```python
from build123d import *

# Parameters (mm, degrees)
F1_DEPTH = 7
F2_R     = 1.6
F3_DEPTH = 25
F4_START = -3.9
F2_R_2   = 3.15
F4_DEPTH = 21.1


with BuildPart() as f1:
    # F0 (on Front) → F1 (new body, symmetric)
    with BuildSketch(Plane.XZ):
        Polygon((-75, 0), (0, 0), (0, 6.4), (-2.7, 6.4), (-2.7, 2.5), (-5.7, 2.5), (-5.7, 5.1), (-4.5, 5.1), (-4.5, 6.4), (-4.5, 7.1), (-7.1, 6.4), (-19.2, 6.4), (-19.2, 6.9), (-31.7, 6.9), (-31.2, 6.4), (-28.7, 3.9), (-47.2, 3.9), (-44.7, 6.4), (-44.2, 6.9), (-56.7, 6.9), (-56.7, 6.4), (-68.1, 6.4), (-70.7, 7.1), (-70.7, 6.4), (-70.7, 5.1), (-69.5, 5.1), (-69.5, 2.5), (-72.5, 2.5), (-72.5, 6.4), (-75, 6.4), align=None)
    extrude(amount=F1_DEPTH, both=True)

    # F2 (on face) → F3 (cut)
    with BuildSketch(Plane(origin=(0, 0, 0), x_dir=(1, 0, 0), z_dir=(0, 0, -1))):
        with Locations((-37.5, 0)):
            Circle(F2_R)
        with Locations((-26.5, 0)):
            Circle(F2_R)
    extrude(amount=-F3_DEPTH, mode=Mode.SUBTRACT)

    # F2 (on face) → F4 (cut)
    with BuildSketch(Plane(origin=(0, 0, 0), x_dir=(1, 0, 0), z_dir=(0, 0, -1)).offset(F4_START)):
        with Locations((-26.5, 0)):
            Circle(F2_R_2)
        with Locations((-26.5, 0)):
            Circle(F2_R, mode=Mode.SUBTRACT)
    extrude(amount=-F4_DEPTH, mode=Mode.SUBTRACT)


solid = f1.part
```
Part model, mm, in its own coordinate system. A direction names the side the tool comes from. Round coordinates to 2 decimals unless told otherwise and drop trailing zeros. Loops run counter-clockwise (first coordinate to the right, second up) from the corner with the lowest first, then second, coordinate; pieces in that order, holes last. Notation, with made-up numbers: (9.5, -30.5) -> (22.5, -30.5) arc R29 cw to (22.5, -5.5) -> close; hole circle Ø5 at (37.5, -24). An arc over 180 degrees is marked (long way). Use CSV: the item, a comma, the result in double quotes. Start each with the question number.
1) Pull direction Z, two halves, no side cores. Call faces 1 (the flat face through (-74, 0, 6.4)), 2 (the flat face through (-69.5, 0, 4)), 3 (the cylindrical face through (-27.68, -1.08, 1.92)): +Z half, -Z half, draft (parallel to the pull), parting line (faces both ways), or undercut.
2) Wall check: L1, parallel to X at y = 0, z = 2.2; L2, parallel to Y at x = -37.5, z = 1.4; L3, parallel to X at y = 0.75, z = 4. Give the ranges that are in metal, low to high. Write a range as [from, to].
3) Drop flat-ended pins along their axis: P1, Ø0.8, axis at x = -73.5, y = 1.5, coming from the +Z side; P2, Ø3, axis at x = -27, y = 2.5, coming from the +Z side; P3, Ø5.5, axis at x = -26.5, y = 0, coming from the +Z side. Give the stop position or say it passes through.
4) Which spindle directions (+Z, -Z, +X, -X, +Y, -Y) get a long thin tool onto all of the face, cutting with end or side? Do faces 4 (the flat face through (-38, -2, 0)), 5 (the flat face through (-70, 0, 5.1)), 6 (the flat face through (-62, 0, 6.4)). Say none if no direction does.
5) Cut at C-C, the plane y = -5. Write the cut outline in (x, z), plus the area to 3 significant figures.
6) Cut at B-B, the plane x = -37.5. Write the cut outline in (y, z), plus the area to 3 significant figures.
7) Cut at A-A, the plane z = 5.75. Write the cut outline in (x, y), plus the area to 3 significant figures.
8) Cut at D-D, the plane x = -45. Write the cut outline in (y, z).
Determined:
1,face 1,"+Z half"
1,face 2,"undercut"
1,face 3,"draft"
2,L1,"x = [-75, -39.1], [-35.9, -28.1], [-24.9, 0]"
2,L2,"y = [-7, -1.6], [1.6, 7]"
2,L3,"x = [-75, -72.5], [-69.5, -47.1], [-23.44, -5.7], [-2.7, 0]"
3,P1,"stops at z = 6.4"
3,P2,"stops at z = 6.9"
3,P3,"stops at z = 3.9"
4,face 4,"-Z, +X, -X, +Y, -Y"
4,face 5,"+Y, -Y"
4,face 6,"+Z, +Y, -Y"
5,outline,"(-75, 0) -> (0, 0) -> (0, 6.4) -> (-2.7, 6.4) -> (-2.7, 2.5) -> (-5.7, 2.5) -> (-5.7, 5.1) -> (-4.5, 5.1) -> (-4.5, 7.1) -> (-7.1, 6.4) -> (-19.2, 6.4) -> (-19.2, 6.9) -> (-31.7, 6.9) -> (-28.7, 3.9) -> (-47.2, 3.9) -> (-44.2, 6.9) -> (-56.7, 6.9) -> (-56.7, 6.4) -> (-68.1, 6.4) -> (-70.7, 7.1) -> (-70.7, 5.1) -> (-69.5, 5.1) -> (-69.5, 2.5) -> (-72.5, 2.5) -> (-72.5, 6.4) -> (-75, 6.4) -> close"
5,area,"434 mm2"
6,outline,"(-7, 0) -> (-1.6, 0) -> (-1.6, 3.9) -> (-7, 3.9) -> close; (1.6, 0) -> (7, 0) -> (7, 3.9) -> (1.6, 3.9) -> close"
6,area,"42.1 mm2"
7,outline,"(-75, -7) -> (-72.5, -7) -> (-72.5, 7) -> (-75, 7) -> close; (-70.7, -7) -> (-45.35, -7) -> (-45.35, 7) -> (-70.7, 7) -> close; (-30.55, -7) -> (-4.5, -7) -> (-4.5, 7) -> (-30.55, 7) -> close; (-2.7, -7) -> (0, -7) -> (0, 7) -> (-2.7, 7) -> close; hole circle Ø6.3 at (-26.5, 0)"
7,area,"761 mm2"
8,outline,"(-7, 0) -> (7, 0) -> (7, 3.9) -> (-7, 3.9) -> close; (-7, 6.1) -> (7, 6.1) -> (7, 6.9) -> (-7, 6.9) -> close"
